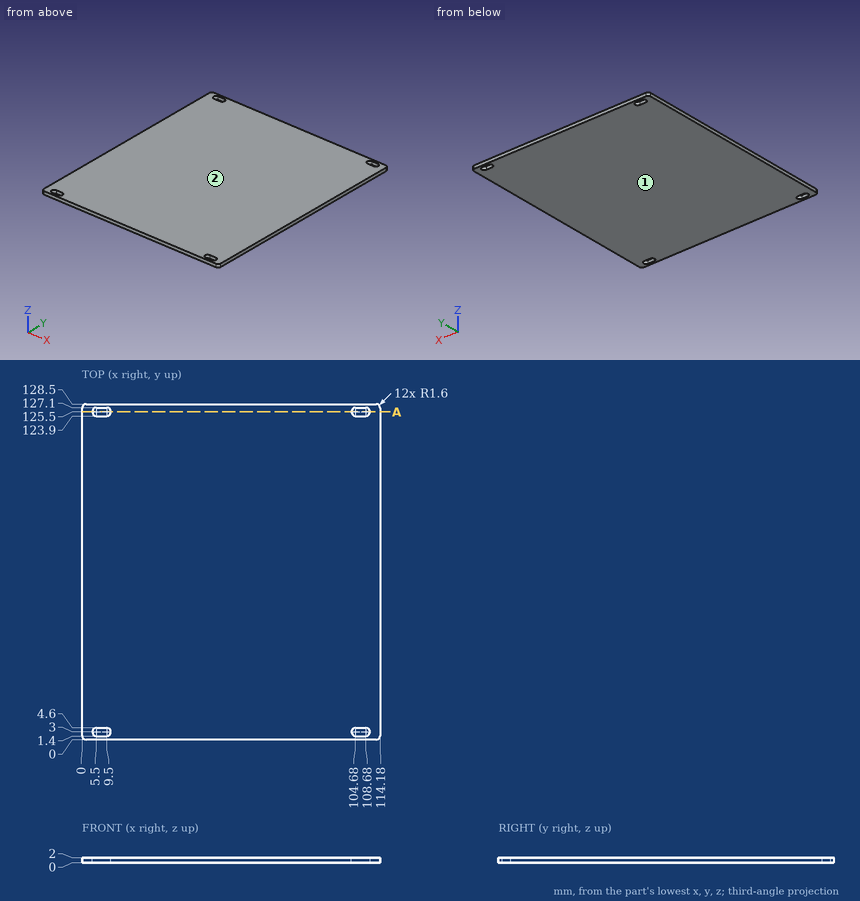
The drawing under review shows one solid part. Ordinate dimensions are in mm from its lowest x, y, z. Round coordinates to 2 decimals unless told otherwise and drop trailing zeros. Loops run counter-clockwise (first coordinate to the right, second up) from the corner with the lowest first, then second, coordinate; pieces in that order, holes last. Notation, with made-up numbers: (79.25, 46.5) - (98.25, 46.5) arc R31 cw to (98.25, 73.5) - close; hole circle Ø5 at (13, 63.5). An arc over 180 degrees is marked (long way). One line per item, written item: value. Start each with the question number.
1) Insertion check: pin 1 Ø5 at (x, y) = (61, 27.5) entering from -Z. The pin has a flat end and moves straight along its axis. Give the tip position at first contact, or say it passes through.
2) To check wall thickness, follow L1, parallel to Y at x = 8, z = 1.6. State the ranges of the line that lie inside material, in increasing order. Write a range as from..to.
3) Consider section A-A on y = 125.5. Give the boundary of the cut face in (x, z), then the cut area to 3 significant figures.
4) Draft analysis for pull direction Z (two halves, no side actions). For the marked faces 1 and 2, state which applies: +Z half, -Z half, draft (parallel to the pull), parting line (faces both ways), or undercut.
Reported:
1. pin 1: stops at z = 0
2. L1: y = 0..1.4, 4.6..123.9, 127.1..128.5
3. outline: (0, 0) - (3.9, 0) - (3.9, 2) - (0, 2) - close; (11.1, 0) - (103.08, 0) - (103.08, 2) - (11.1, 2) - close; (110.28, 0) - (114.18, 0) - (114.18, 2) - (110.28, 2) - close
3. area: 200 mm^2
4. face 1: -Z half
4. face 2: +Z half
